from build123d import *

# Parameters (mm, degrees)
FILLET1_R   = 0.2
FILLET2_R   = 0.5
HEX_2_DEPTH = 2


with BuildPart() as part:
    # BodySke → Base-Revolve (revolve)
    with BuildSketch(Plane.XY, mode=Mode.PRIVATE) as base_revolve_sk:
        Polygon((0, 0), (0, 4.25), (3.5, 4.25), (3.5, 2.5), (33.055, 2.5), (33.5, 2.055), (33.5, 0), align=None)
    revolve(base_revolve_sk.sketch.rotate(Axis((-31.75, 0, 0), (1, 0, 0)), 90), axis=Axis((-31.75, 0, 0), (1, 0, 0)))

    # Fillet1
    fillet1_edges = [part.edges().sort_by_distance(p)[0] for p in [
        (3.5, 0, -2.5),
    ]]
    fillet(fillet1_edges, radius=FILLET1_R)

    # Fillet2
    fillet2_edges = [part.edges().sort_by_distance(p)[0] for p in [
        (0, 0, -4.25),
    ]]
    fillet(fillet2_edges, radius=FILLET2_R)

    # HexSke → Hex 2 (cut)
    with BuildSketch(Plane(origin=(0, 0, 0), x_dir=(0, 0.500000000000001, 0.866025403784438), z_dir=(-1, 0, 0))):
        Polygon((1.154700538, 2), (-1.154700538, 2), (-2.309401077, 0), (-1.154700538, -2), (1.154700538, -2), (2.309401077, 0), align=None)
    extrude(amount=-HEX_2_DEPTH, mode=Mode.SUBTRACT)

    # PilotSke → Hex-PreBroach (revolve, cut)
    with BuildSketch(Plane.XY, mode=Mode.PRIVATE) as hex_prebroach_sk:
        Polygon((0, 2), (2, 2), (2.433012702, 1.25), (4, 1.25), (4.721687836, 0), (0, 0), align=None)
    revolve(hex_prebroach_sk.sketch.rotate(Axis((0, 0, 0), (1, 0, 0)), 90), axis=Axis((0, 0, 0), (1, 0, 0)), mode=Mode.SUBTRACT)


solid = part.part
Can you work these out from the model? Positions are in its coordinate system, mm. A direction names the side the tool comes from. Coordinates: 2 decimals unless noted, no trailing zeros. Loops run counter-clockwise (first coordinate to the right, second up) from the corner with the lowest first, then second, coordinate; pieces in that order, holes last. Notation, with made-up numbers: (45, 54.5) - (69, 54.5) arc R15 cw to (69, 73.5) - close; hole circle Ø1 at (-27.75, 2). An arc over 180 degrees is marked (long way). Put each result on its own line as item: value. Start each with the question number.
Item 1: For pin 1 (5 mm diameter, centred on x = 26.5, y = -3, fed in from -Z); pin 2 (0.5 mm diameter, centred on y = 1, z = -1.5, fed in from -X); pin 3 (0.6 mm diameter, centred on x = 1.5, y = -0.5, fed in from +Z); pin 4 (1.5 mm diameter, centred on x = 7, z = -3.5, fed in from -Y), each with a flat end and sliding along its axis, tell me the tip position at first contact or that it passes through.
Item 2: If we mould it in two halves opening along Y, with no side actions, what happens to faces 1 (the face through (1, 0, -2)), 2 (the face through (3.5, 3, 0)), 3 (the face through (2.021, -4.214, -0.553)), 4 (the face through (0.986, 1.724, 1.014))? For each: +Y half, -Y half, draft (parallel to the pull), parting line (faces both ways), or undercut.
Item 3: Suppose I cut it at A-A (x = 7). Please give me the cut outline in (y, z), and give its area (3 significant figures).
Item 4: Which directions (+Z, -Z, +X, -X, +Y, -Y) give clear straight access to the entire face, cutting with the end or side of a thin tool? Please do faces 5 (the face through (3.23, -0.05, -1.25)), 6 (the face through (33.5, 0, 0)), 7 (the face through (18.6, -0.1, -2.5)).
Item 5: If I drill on line 1 along Y through (x, z) = (3.7, 0); line 2 along Y through (x, z) = (2.85, 0); line 3 along Y through (x, z) = (7.5, 1.5), over which ranges is the centre line in solid material (lowest first)?
Here are the results:
1. pin 1: z = -2.45
1. pin 2: x = 2
1. pin 3: z = 4.25
1. pin 4: through
2. face 1: undercut
2. face 2: draft
2. face 3: parting line
2. face 4: undercut
3. outline: circle Ø5 at (0, 0)
3. area: 19.6 mm²
4. face 5: -X
4. face 6: +Z, -Z, +X, +Y, -Y
4. face 7: +X
5. line 1: -2.5 to -1.25, 1.25 to 2.5
5. line 2: -4.25 to -1.25, 1.25 to 4.25
5. line 3: -2 to 2
